```python
from build123d import *

# Parameters (mm, degrees)
SKETCH1_R           = 1.75
BOSS_EXTRUDE1_DEPTH = 60
SKETCH2_R           = 1.5
CUT_EXTRUDE1_DEPTH  = 60


with BuildPart() as part:
    # Sketch1 → Boss-Extrude1 (new body)
    with BuildSketch(Plane(origin=(0, 0, 0), x_dir=(1, 0, 0), z_dir=(0, 1, 0))):
        with BuildLine():
            Line((8.14420001, -1.125), (8.14420001, -2.125))
            Line((8.14420001, -2.125), (2.459039447, -2.125))
            ThreePointArc((2.459039447, -2.125), (-3.25, 0), (2.459039447, 2.125))
            Line((2.459039447, 2.125), (8.14420001, 2.125))
            Line((8.14420001, 2.125), (8.14420001, 1.125))
            Line((8.14420001, 1.125), (3.14420001, 1.125))
            Line((3.14420001, 1.125), (3.14420001, -1.125))
            Line((3.14420001, -1.125), (8.14420001, -1.125))
        make_face()
        with Locations(Location((0, 0, 0), (0, 0, 270))):
            Circle(SKETCH1_R, mode=Mode.SUBTRACT)
    extrude(amount=BOSS_EXTRUDE1_DEPTH)

    # Sketch2 → Cut-Extrude1 (cut)
    with BuildSketch(Plane.XY.offset(2.125)):
        with Locations((5.64420001, 45)):
            Circle(SKETCH2_R)
        with Locations((5.64420001, 15)):
            Circle(SKETCH2_R)
    extrude(amount=-CUT_EXTRUDE1_DEPTH, mode=Mode.SUBTRACT)


solid = part.part
```
The listing builds one solid part. Answer for the finished solid, in the listing's coordinates (mm). A direction names the side the tool comes from. Round coordinates to 2 decimals unless told otherwise and drop trailing zeros. Loops run counter-clockwise (first coordinate to the right, second up) from the corner with the lowest first, then second, coordinate; pieces in that order, holes last.
Q1. For a pull along Y with two mould halves and no side action, classify faces 1 (the face through (5.319, 43.536, -1.618)), 2 (the face through (2.5, 60, 0)), 3 (the face through (-3.25, 29.58, 0.11)), 4 (the face through (4.539, 16.014, -1.618)) as released by +Y, released by -Y, zero draft, split by the parting line, or undercut.
Q2. Section B-B, the plane x = 0 is taken. Determine the outline of the cut face in (y, z).
Q3. Given pin 1 Ø1.7 at (x, y) = (5, 18.5) entering from -Z (3 decimals); pin 2 Ø6.5 at (x, y) = (5.5, 27.5) entering from +Z; pin 3 Ø4 at (x, y) = (5, 23) entering from +Z (3 decimals), each flat-ended and moving along its own axis, determine where each tip first touches the part or whether it passes through.
Q4. Find the intervals of material crossed by line 1 (Y direction, x = 4.75, z = 1.5); line 2 (Z direction, x = 6.5, y = 41) (3 decimals); line 3 (X direction, y = 57, z = 1.5), in increasing order.
Q5. Section D-D, the plane y = 5 is taken. Determine the outline of the cut face in (x, z) (3 decimals).
Q6. Section C-C, the plane z = 0 is taken. Determine the outline of the cut face in (x, y), then the cut area to 3 significant figures.
Q7. Section A-A, the plane y = 45 is taken. Determine the outline of the cut face in (x, z) (3 decimals), then the cut area to 3 significant figures.
Q8. Which of the six approach directions +Z, -Z, +X, -X, +Y, -Y give full straight-line access (tool end or side, diameter ignored) to faces 5 (the face through (5, 30, 2.125)), 6 (the face through (4.539, 16.014, 1.632)), 7 (the face through (5, 30, -2.125)), 8 (the face through (6, 30, -1.125))?
Completed:
1. face 1: undercut
1. face 2: released by +Y
1. face 3: zero draft
1. face 4: undercut
2. outline: (0, -3.25) - (60, -3.25) - (60, -1.75) - (0, -1.75) - close; (0, 1.75) - (60, 1.75) - (60, 3.25) - (0, 3.25) - close
3. pin 1: stops at z = -2.125
3. pin 2: stops at z = 2.35
3. pin 3: stops at z = 2.125
4. line 1: y = 0 to 13.8, 16.2 to 43.8, 46.2 to 60
4. line 2: z = -2.125 to -1.125, 1.125 to 2.125
4. line 3: x = -2.88 to -0.9, 0.9 to 8.14
5. outline: (2.459, -2.125) - (8.144, -2.125) - (8.144, -1.125) - (3.144, -1.125) - (3.144, 1.125) - (8.144, 1.125) - (8.144, 2.125) - (2.459, 2.125) arc R3.25 ccw (long way) to start; hole circle Ø3.5 at (0, 0)
6. outline: (-3.25, 0) - (-1.75, 0) - (-1.75, 60) - (-3.25, 60) - close; (1.75, 0) - (3.14, 0) - (3.14, 60) - (1.75, 60) - close
6. area: 174 mm2
7. outline: (2.459, -2.125) - (4.144, -2.125) - (4.144, -1.125) - (3.144, -1.125) - (3.144, 1.125) - (4.144, 1.125) - (4.144, 2.125) - (2.459, 2.125) arc R3.25 ccw (long way) to start; (7.144, -2.125) - (8.144, -2.125) - (8.144, -1.125) - (7.144, -1.125) - close; (7.144, 1.125) - (8.144, 1.125) - (8.144, 2.125) - (7.144, 2.125) - close; hole circle Ø3.5 at (0, 0)
7. area: 28.2 mm2
8. face 5: +Z, +X, +Y, -Y
8. face 6: +Z, -Z
8. face 7: -Z, +X, +Y, -Y
8. face 8: +X, +Y, -Y
